```python
from build123d import *

# Parameters (mm, degrees)
SKETCH1_W                     = 254
SKETCH1_H                     = 98.425
SKETCH1_R                     = 6.35
BOSS_EXTRUDE1_DEPTH           = 3.175
TAP_DRILL_FOR_1_4_HELICOIL2_D = 6.7564
FILLET1_R                     = 3.175


with BuildPart() as part:
    # Sketch1 → Boss-Extrude1 (new body)
    # profile 1 of 2: a face of its own
    with BuildSketch(Plane(origin=(0, 0, 0), x_dir=(1, 0, 0), z_dir=(0, 1, 0))):
        Rectangle(SKETCH1_W, SKETCH1_H)
        with Locations((-114.3, 36.5125)):
            Circle(SKETCH1_R, mode=Mode.SUBTRACT)
    # profile 2 of 2: a face of its own
    with BuildSketch(Plane(origin=(0, 0, 0), x_dir=(1, 0, 0), z_dir=(0, 1, 0))):
        with Locations((-114.3, 36.5125)):
            Circle(SKETCH1_R)
    extrude(amount=BOSS_EXTRUDE1_DEPTH)

    # Tap Drill for 1/4 Helicoil2 (through all)
    with Locations(Plane(origin=(0, 0, 0), x_dir=(-1, 0, 0), z_dir=(0, -1, 0))):
        with Locations((-114.3, 36.5125), (-114.3, 11.1125), (-114.3, -14.2875), (-57.15, -39.6875), (0, -39.6875), (57.15, -39.6875), (114.3, -14.2875), (114.3, 11.1125), (114.3, 36.5125), (114.3, -39.6875), (-114.3, -39.6875)):
            Hole(TAP_DRILL_FOR_1_4_HELICOIL2_D / 2)

    # Fillet1
    fillet1_edges = [part.edges().sort_by_distance(p)[0] for p in [
        (-127, 1.5875, 49.2125),
        (-127, 1.5875, -49.2125),
        (127, 1.5875, -49.2125),
        (127, 1.5875, 49.2125),
    ]]
    fillet(fillet1_edges, radius=FILLET1_R)


solid = part.part
```
Could you check a few things on this model? Use its own coordinates, in mm. Give positions to 0.01 mm unless a question says otherwise; leave off trailing zeros. Order: outer loops, then holes, each group sorted by start corner. A loop starts at its lowest first (then second) coordinate and runs counter-clockwise, first axis right, second up.
Q1. Suppose I cut it at A-A, the plane x = 0. Write out the boundary of the cut face in (y, z) (1 decimal), and give its area (3 significant figures).
Q2. Suppose I cut it at B-B, the plane x = 114.3. Write out the boundary of the cut face in (y, z) (1 decimal).
Q3. We'd pull the mould along X, two halves only. Please class faces 1 (the flat face through (-2, 0, -1)), 2 (the cylindrical face through (-111.18, 1.61, -9.82)): +X half, -X half, draft (parallel to the pull), parting line (faces both ways), or undercut.
Q4. If I drill on line 1 along Z through (x, y) = (-114.3, 2.3); line 2 along X through (y, z) = (2.3, 40.5); line 3 along X through (y, z) = (1.35, -14), over which ranges is the centre line in solid material (lowest first)?
Q5. Suppose I cut it at C-C, the plane y = 1.1. Count the separate pieces of the cut face and the enclosed holes in it, and give its area (3 significant figures).
Solution:
1. outline: (0, -49.2) - (3.2, -49.2) - (3.2, 36.3) - (0, 36.3) - close; (0, 43.1) - (3.2, 43.1) - (3.2, 49.2) - (0, 49.2) - close
1. area: 291 mm2
2. outline: (0, -49.2) - (3.2, -49.2) - (3.2, -39.9) - (0, -39.9) - close; (0, -33.1) - (3.2, -33.1) - (3.2, -14.5) - (0, -14.5) - close; (0, -7.7) - (3.2, -7.7) - (3.2, 10.9) - (0, 10.9) - close; (0, 17.7) - (3.2, 17.7) - (3.2, 36.3) - (0, 36.3) - close; (0, 43.1) - (3.2, 43.1) - (3.2, 49.2) - (0, 49.2) - close
3. face 1: draft
3. face 2: undercut
4. line 1: z = -49.21 to -39.89, -33.13 to -14.49, -7.73 to 10.91, 17.67 to 36.31, 43.07 to 49.21
4. line 2: x = -127 to -117.58, -111.02 to -60.43, -53.87 to -3.28, 3.28 to 53.87, 60.43 to 111.02, 117.58 to 127
4. line 3: x = -127 to -116.05, -112.55 to 112.55, 116.05 to 127
5. separate pieces: 1
5. enclosed holes: 11
5. area: 24,600 mm2
